Can you work these out from the model? Positions are in its coordinate system, mm. A direction names the side the tool comes from. Round coordinates to 2 decimals unless told otherwise and drop trailing zeros. Order: outer loops, then holes, each group sorted by start corner. A loop starts at its lowest first (then second) coordinate and runs counter-clockwise, first axis right, second up.
Q1. For faces 1 (the face through (101.6, -3, 56)), 2 (the face through (98.38, -197, 57.71)), 3 (the face through (-95.25, -3, 56)), which set-ups out of +Z, -Z, +X, -X, +Y, -Y let a thin tool reach every point of the face, with its end or its side?
Q2. If we section it at B-B (z = 57.15): Please give me the cut outline in (x, y), plus the area to 3 significant figures.
Q3. If we section it at D-D (z = 27.5): Please give me the cut outline in (x, y), plus the area to 3 significant figures.
Q4. If we section it at A-A (x = -57): Please give me the cut outline in (y, z).
Q5. We'd pull the mould along Y, two halves only. Please class faces 4 (the face through (-1, -215.9, 56)), 5 (the face through (97, 1, 0)), 6 (the face through (-1, 209.55, 56)), 7 (the face through (-1, 215.9, 56)): pulls with the +Y half, pulls with the -Y half, needs draft (parallel to the pull), parting line crosses it, or undercut.
Q6. If I drill on line 1 (Y direction, x = 98.75, z = 57.15); line 2 (Y direction, x = 32, z = 35); line 3 (X direction, y = 150.5, z = 89.5), over which ranges is the centre line in solid material (lowest first)?
Q7. If we section it at C-C (y = 55.5): Please give me the cut outline in (x, z).
from build123d import *

# Parameters (mm, degrees)
SKETCH1_W              = 203.2
SKETCH1_H              = 431.8
SKETCH1_W_2            = 190.5
SKETCH1_H_2            = 419.1
BOSS_EXTRUDE4_DEPTH    = 114.3
CUT_EXTRUDE3_START     = -101.6
CUT_EXTRUDE3_OUTLINE_R = 25.313218752
CUT_EXTRUDE3_DEPTH     = 203.2


# Read off the part's stored shape, not the designer's step: Cut-Extrude3
with BuildPart() as part:
    # Sketch1 → Boss-Extrude4 (new body)
    with BuildSketch(Plane.XY):
        Rectangle(SKETCH1_W, SKETCH1_H)
        Rectangle(SKETCH1_W_2, SKETCH1_H_2, mode=Mode.SUBTRACT)
    extrude(amount=BOSS_EXTRUDE4_DEPTH)

    # Cut-Extrude3 outline → Cut-Extrude3 (cut)
    with BuildSketch(Plane(origin=(0, 0, 0), x_dir=(0, 0, -1), z_dir=(1, 0, 0)).offset(CUT_EXTRUDE3_START)):
        with BuildLine():
            Line((-82.252642197, -53.975), (-82.55, -171.608124436))
            ThreePointArc((-82.55, -171.608124436), (-57.15, -197.008124436), (-31.75, -171.608124436))
            Line((-31.75, -171.608124436), (-32.047357803, -53.975))
            ThreePointArc((-32.047357803, -53.975), (-57.15, -28.872357803), (-82.252642197, -53.975))
        make_face()
        with Locations((-57.15, 137.213144343)):
            Circle(CUT_EXTRUDE3_OUTLINE_R)
    extrude(amount=CUT_EXTRUDE3_DEPTH, mode=Mode.SUBTRACT)


solid = part.part
Solution:
1. face 1: +Z, -Z, +X, +Y, -Y
1. face 2: +X, -X
1. face 3: +Z, -Z
2. outline: (-101.6, -215.9) - (101.6, -215.9) - (101.6, -197.01) - (95.25, -197.01) - (95.25, -209.55) - (-95.25, -209.55) - (-95.25, -197.01) - (-101.6, -197.01) - close; (-101.6, -28.87) - (-95.25, -28.87) - (-95.25, 111.9) - (-101.6, 111.9) - close; (-101.6, 162.53) - (-95.25, 162.53) - (-95.25, 209.55) - (95.25, 209.55) - (95.25, 162.53) - (101.6, 162.53) - (101.6, 215.9) - (-101.6, 215.9) - close; (95.25, -28.87) - (101.6, -28.87) - (101.6, 111.9) - (95.25, 111.9) - close
2. area: 5,120 mm2
3. outline: (-101.6, -215.9) - (101.6, -215.9) - (101.6, 215.9) - (-101.6, 215.9) - close; hole (-95.25, -209.55) - (95.25, -209.55) - (95.25, 209.55) - (-95.25, 209.55) - close
3. area: 7,900 mm2
4. outline: (-215.9, 0) - (-209.55, 0) - (-209.55, 114.3) - (-215.9, 114.3) - close; (209.55, 0) - (215.9, 0) - (215.9, 114.3) - (209.55, 114.3) - close
5. face 4: pulls with the -Y half
5. face 5: needs draft
5. face 6: undercut
5. face 7: pulls with the +Y half
6. line 1: y = -215.9 to -197.01, -28.87 to 111.9, 162.53 to 215.9
6. line 2: y = -215.9 to -209.55, 209.55 to 215.9
6. line 3: x = -101.6 to -95.25, 95.25 to 101.6
7. outline: (-101.6, 0) - (-95.25, 0) - (-95.25, 114.3) - (-101.6, 114.3) - close; (95.25, 0) - (101.6, 0) - (101.6, 114.3) - (95.25, 114.3) - close
